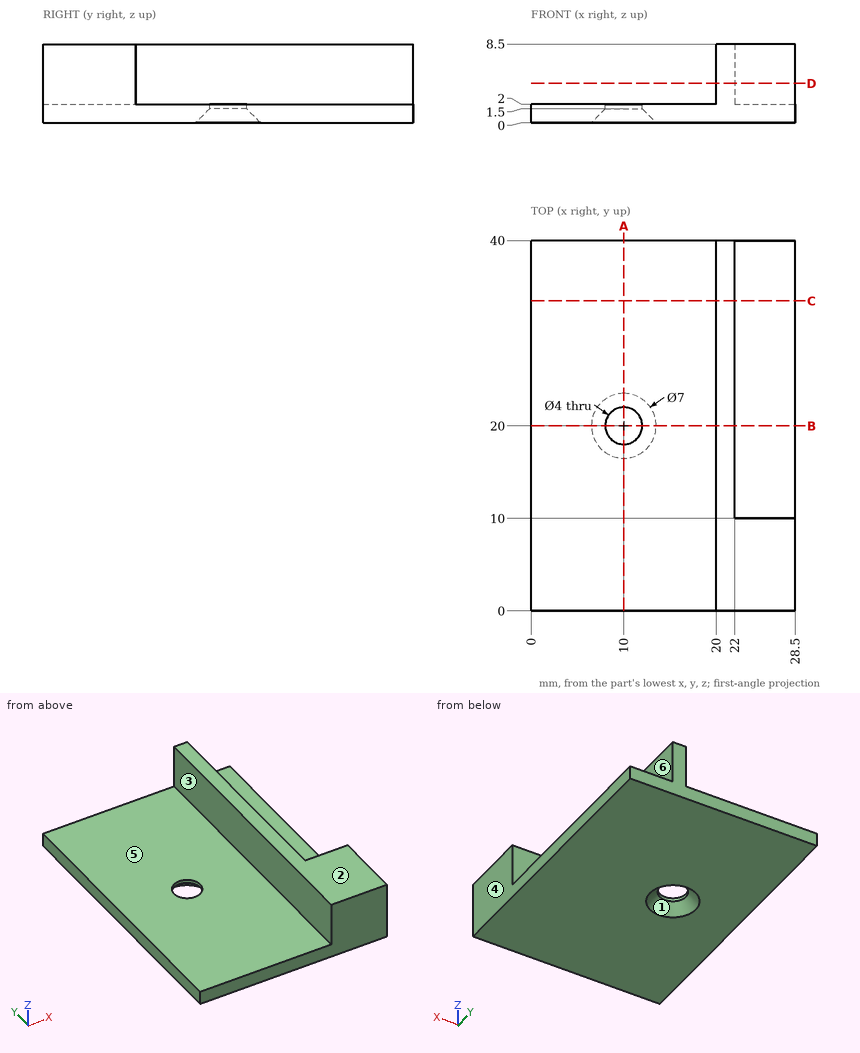
Here's the drawing with two shaded views (mm, measured from the low corner). I have some questions. A direction names the side the tool comes from. Give positions to 0.01 mm unless a question says otherwise; leave off trailing zeros. Loops run counter-clockwise (first coordinate to the right, second up) from the corner with the lowest first, then second, coordinate; pieces in that order, holes last. Notation, with made-up numbers: M -36.5,-5 L -2.5,-5 A28 ccw -2.5,16 Z; hole C 63,24.5 d5. An arc over 180 degrees is marked long. Use one line per item in the form item = value. Start each with the question number.
Q1. I need wall thicknesses on line 1 along X through (y, z) = (20, 1.8); line 2 along Y through (x, z) = (10, 1.7); line 3 along Z through (x, y) = (25.5, 28.5). Which ranges of each line are inside material? Lowest first, please.
Q2. If we section it at A-A (x = 10): Write out the boundary of the cut face in (y, z), then the cut area to 4 significant figures.
Q3. If we section it at B-B (y = 20): Write out the boundary of the cut face in (x, z).
Q4. If we section it at D-D (z = 4.25): Write out the boundary of the cut face in (x, y), then the cut area to 3 significant figures.
Q5. Will these pins go through, and if not, where does the flat tip stop? pin 1 Ø3 at (y, z) = (23, 4.5) entering from +X; pin 2 Ø2 at (x, y) = (24.5, 30.5) entering from +Z; pin 3 Ø4.5 at (x, y) = (10, 20) entering from -Z.
Q6. Thinking about a two-plate mould opening in X: for the marked faces 1, 2 and 3, which applies, +X half, -X half, draft (parallel to the pull), parting line (faces both ways), or undercut?
Q7. If we section it at C-C (y = 33.5): Write out the boundary of the cut face in (x, z).
Q8. Which directions (+Z, -Z, +X, -X, +Y, -Y) give clear straight access to the entire face, cutting with the end or side of a thin tool? Please do the marked faces 4, 5 and 6.
Taken from the geometry:
q1.line_1 = 0 to 8, 12 to 28.5
q1.line_2 = 0 to 18, 22 to 40
q1.line_3 = 0 to 2
q2.outline = M 0,0 L 16.5,0 L 18,1.5 L 18,2 L 0,2 Z; M 22,1.5 L 23.5,0 L 40,0 L 40,2 L 22,2 Z
q2.area = 69.75 mm^2
q3.outline = M 0,0 L 6.5,0 L 8,1.5 L 8,2 L 0,2 Z; M 12,1.5 L 13.5,0 L 28.5,0 L 28.5,2 L 22,2 L 22,8.5 L 20,8.5 L 20,2 L 12,2 Z
q4.outline = M 20,0 L 28.5,0 L 28.5,10 L 22,10 L 22,40 L 20,40 Z
q4.area = 145 mm^2
q5.pin_1 = 22
q5.pin_2 = 2
q5.pin_3 = 1.25
q6.face_1 = undercut
q6.face_2 = draft
q6.face_3 = -X half
q7.outline = M 0,0 L 28.5,0 L 28.5,2 L 22,2 L 22,8.5 L 20,8.5 L 20,2 L 0,2 Z
q8.face_4 = +Z, -Z, +X, +Y, -Y
q8.face_5 = +Z, -X, +Y, -Y
q8.face_6 = +Z, +X, +Y
